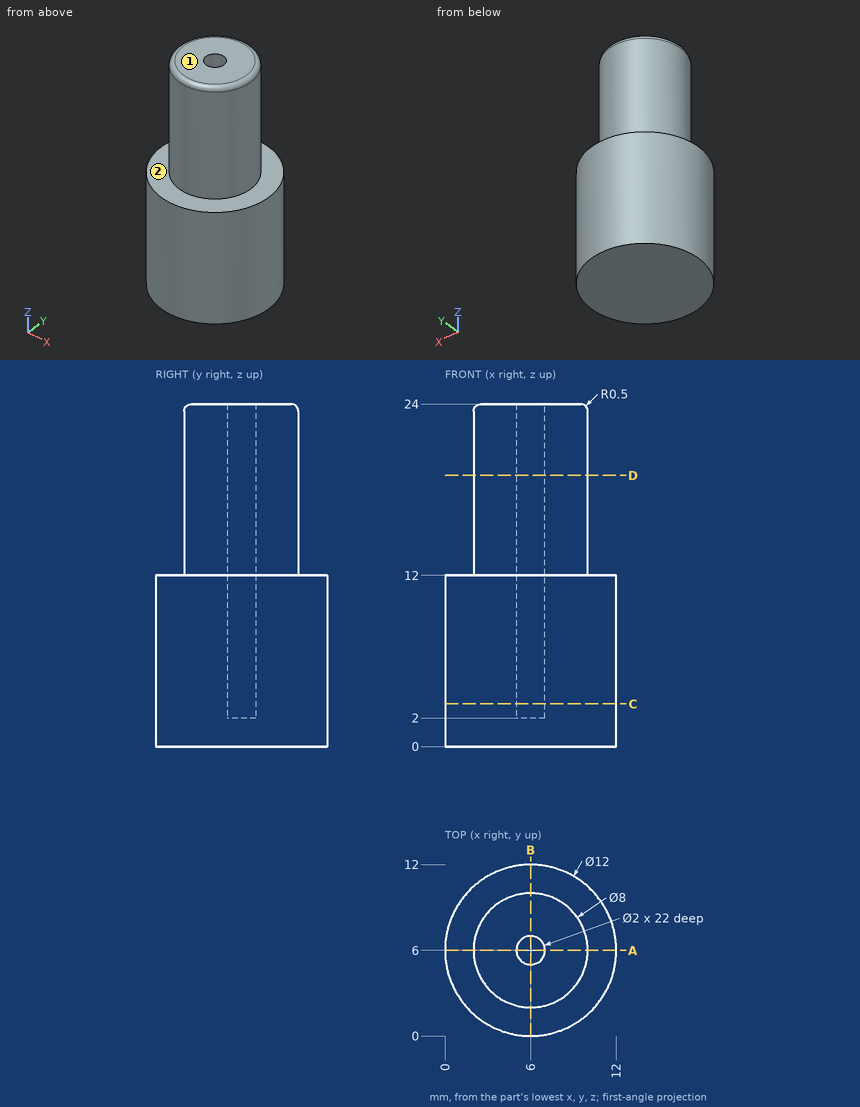
Part print with two shaded views. Sizes in mm from the minimum x, y, z corner. A direction names the side the tool comes from. Round coordinates to 2 decimals unless told otherwise and drop trailing zeros. Write each loop counter-clockwise with the first axis right and the second up, starting at its lowest first coordinate (ties: lowest second). Pieces come first, ordered by that corner, then holes. Notation, with made-up numbers: M -8.75,-32 L 0.25,-32 A14 cw 0.25,-13 Z; hole C 18.25,-9 d7. An arc over 180 degrees is marked long. Answer as CSV lines item,"result". Start each with the question number.
1) Which spindle directions (+Z, -Z, +X, -X, +Y, -Y) get a long thin tool onto all of the face, cutting with end or side? Do the marked faces 1 and 2. Say none if no direction does.
2) Drill centre lines: L1, parallel to Y at x = 6, z = 19; L2, parallel to Z at x = 4.75, y = 2; L3, parallel to X at y = 6.75, z = 20.75. Where is each one in solid material? Low to high.
3) Band-saw the part on D-D (z = 19). List the corners of the cut face in (x, y), then the cut area to 3 significant figures.
4) Band-saw the part on C-C (z = 3). List the corners of the cut face in (x, y), then the cut area to 3 significant figures.
5) Drop flat-ended pins along their axis: pin 1 (6 mm diameter, centred on x = 2, z = 6.5, fed in from +Y); pin 2 (4 mm diameter, centred on x = 5, z = 19.5, fed in from -Y); pin 3 (2 mm diameter, centred on y = 2, z = 18.5, fed in from -X). Give the stop position or say it passes through.
6) Band-saw the part on A-A (y = 6). List the corners of the cut face in (x, z), then the cut area to 3 significant figures.
Worked out:
1,face 1,"+Z, +X, -X, +Y, -Y"
1,face 2,"+Z"
2,L1,"2 to 5, 7 to 10"
2,L2,"0 to 12"
2,L3,"2.07 to 5.34, 6.66 to 9.93"
3,outline,"C 6,6 d8; hole C 6,6 d2"
3,area,"47.1 mm²"
4,outline,"C 6,6 d12; hole C 6,6 d2"
4,area,"110 mm²"
5,pin 1,"y = 11.92"
5,pin 2,"y = 2"
5,pin 3,"x = 3.35"
6,outline,"M 0,0 L 12,0 L 12,12 L 10,12 L 10,23.5 A0.5 ccw 9.5,24 L 7,24 L 7,2 L 5,2 L 5,24 L 2.5,24 A0.5 ccw 2,23.5 L 2,12 L 0,12 Z"
6,area,"196 mm²"
